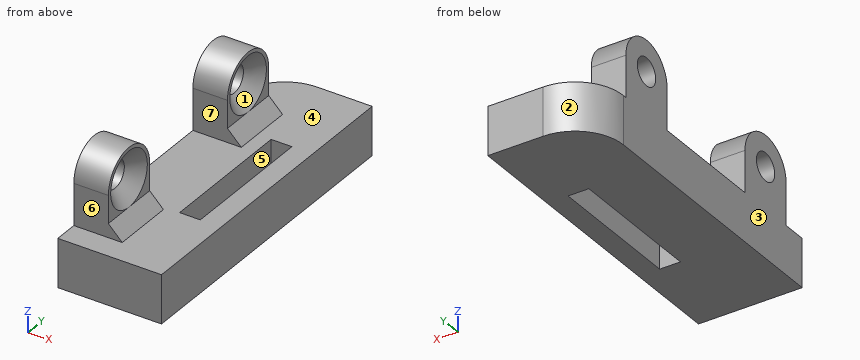
from build123d import *

# Parameters (mm, degrees)
BOSS_EXTRUDE1_DEPTH = 7
SKETCH2_R           = 2
BOSS_EXTRUDE2_DEPTH = 5
CHAMFER1_SIZE       = 2
CHAMFER2_SIZE       = 2
SKETCH3_W           = 3
SKETCH3_H           = 20
CUT_EXTRUDE1_DEPTH  = 38.619808612


with BuildPart() as part:
    # Sketch1 → Boss-Extrude1 (new body)
    with BuildSketch(Plane.XY):
        with BuildLine():
            Line((22, 21), (14, 21))
            ThreePointArc((14, 21), (9.050252532, 18.949747468), (7, 14))
            Line((7, 14), (7, -25))
            Line((7, -25), (22, -25))
            Line((22, -25), (22, 21))
        make_face()
    extrude(amount=BOSS_EXTRUDE1_DEPTH)

    # Sketch2 → Boss-Extrude2 (add)
    with BuildSketch(Plane.ZY.offset(-7)):
        with BuildLine():
            Line((7, 13.5), (13, 13.5))
            ThreePointArc((13, 13.5), (17.5, 9), (13, 4.5))
            Line((13, 4.5), (7, 4.5))
            Line((7, 4.5), (7, 13.5))
        make_face()
        with Locations(Location((13, 9, 0), (0, 0, 270))):
            Circle(SKETCH2_R, mode=Mode.SUBTRACT)
    boss_extrude2 = extrude(amount=-BOSS_EXTRUDE2_DEPTH)

    # Mirror1: Boss-Extrude2 across plane
    add(boss_extrude2.mirror(Plane.ZX.offset(-4)))

    # Chamfer1
    chamfer1_edges = [part.edges().sort_by_distance(p)[0] for p in [
        (12, 11, 13),
        (12, -19, 13),
    ]]
    chamfer(chamfer1_edges, length=CHAMFER1_SIZE)

    # Chamfer2
    chamfer2_edges = [part.edges().sort_by_distance(p)[0] for p in [
        (12, 9, 7),
        (12, -17, 7),
    ]]
    chamfer(chamfer2_edges, length=CHAMFER2_SIZE - 0.0001)  # a hair under: the kernel refuses the full size

    # Sketch3 → Cut-Extrude1 (cut, through all)
    with BuildSketch(Plane(origin=(0, 0, 0), x_dir=(-1, 0, 0), z_dir=(0, 0, -1))):
        with Locations((-17.5, -2)):
            Rectangle(SKETCH3_W, SKETCH3_H)
    extrude(amount=-CUT_EXTRUDE1_DEPTH, mode=Mode.SUBTRACT)


solid = part.part
Verification items for the finished model (mm, model axes). Face numbers are marked on the shaded views. A direction names the side the tool comes from. Coordinates: 2 decimals unless noted, no trailing zeros. Order: outer loops, then holes, each group sorted by start corner. A loop starts at its lowest first (then second) coordinate and runs counter-clockwise, first axis right, second up.
1. Sectioned sample at D-D, the plane z = 5.75. Record the cut outline in (x, y).
Results found:
outline: (7, -25) - (22, -25) - (22, 21) - (14, 21) arc R7 ccw to (7, 14) - close; hole (16, -12) - (19, -12) - (19, 8) - (16, 8) - close
2. Sectioned sample at A-A, the plane x = 16.75. Record the cut outline in (y, z), and give its area (3 significant figures).
Results found:
outline: (-25, 0) - (-12, 0) - (-12, 7) - (-25, 7) - close; (8, 0) - (21, 0) - (21, 7) - (8, 7) - close
area: 182 mm2
3. Set-up check for the marked faces 4, 5, 6 and 7: record each of +Z, -Z, +X, -X, +Y, -Y from which the full face is reachable in a straight line by a thin tool's end or side.
Results found:
face 4: +Z, +X
face 5: +Z, -Z
face 6: +Z, +X, -X, -Y
face 7: +Z, +X, -X
4. Go/stop test with flat-tipped pins: pin 1 Ø1 at (x, y) = (14.5, 16) entering from +Z; pin 2 Ø3 at (x, z) = (10.5, 10) entering from -Y; pin 3 Ø4.5 at (y, z) = (-18.5, 13.5) entering from +X. Record where each tip stops, or that it passes through.
Results found:
pin 1: stops at z = 7
pin 2: stops at y = -21.5
pin 3: stops at x = 11.83
5. Sectioned sample at B-B, the plane z = 8.5. Record the cut outline in (x, y).
Results found:
outline: (7, -21.5) - (12.5, -21.5) - (12.5, -12.5) - (7, -12.5) - close; (7, 4.5) - (12.5, 4.5) - (12.5, 13.5) - (7, 13.5) - close
6. Release check for a two-part mould opening along Y. For the marked faces 1, 2 and 3 record: +Y half, -Y half, draft (parallel to the pull), parting line (faces both ways), or undercut.
Results found:
face 1: undercut
face 2: +Y half
face 3: draft
7. Scan lines: line 1 (Z direction, x = 9.2, y = -17); line 2 (Y direction, x = 17, z = 3.5); line 3 (Y direction, x = 9.25, z = 9). Record each from-to range of solid material in increasing order.
Results found:
line 1: z = 0 to 11, 15 to 17.5
line 2: y = -25 to -12, 8 to 21
line 3: y = -21.5 to -12.5, 4.5 to 13.5
